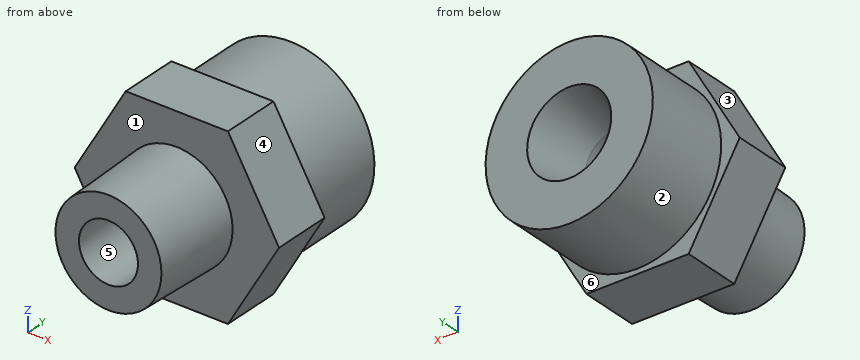
```python
from build123d import *

# Parameters (mm, degrees)
SKETCH1_R           = 9
BOSS_EXTRUDE1_DEPTH = 9.525
SKETCH4_R           = 3.175
CUT_EXTRUDE1_DEPTH  = 3.175
SKETCH5_R           = 3.175
CUT_EXTRUDE2_DEPTH  = 15.224011389
CUT_EXTRUDE2_DRAFT  = 12
BOSS_EXTRUDE3_START = 6.35
SKETCH6_R           = 3.175
BOSS_EXTRUDE3_DEPTH = 6.35
SKETCH7_R           = 6
BOSS_EXTRUDE4_DEPTH = 9.525
BOSS_EXTRUDE4_TAPER = 1.79
SKETCH8_R           = 3.175
CUT_EXTRUDE3_DEPTH  = 30.272053652


with BuildPart() as part:
    # Sketch1 → Boss-Extrude1 (new body)
    with BuildSketch(Plane(origin=(0, 0, 0), x_dir=(1, 0, 0), z_dir=(0, 1, 0))):
        with Locations(Location((0, 0, 0), (0, 0, 90))):
            Circle(SKETCH1_R)
    extrude(amount=BOSS_EXTRUDE1_DEPTH)

    # Sketch4 → Cut-Extrude1 (cut)
    with BuildSketch(Plane.XZ):
        with Locations(Location((0, 0, 0), (0, 0, 270))):
            Circle(SKETCH4_R)
    extrude(amount=-CUT_EXTRUDE1_DEPTH, mode=Mode.SUBTRACT)


with BuildPart() as cut_extrude2_tool:
    # Sketch5 → Cut-Extrude2 (with draft: the straight prism first)
    with BuildSketch(Plane(origin=(0, 3.175, 0), x_dir=(-1, 0, 0), z_dir=(0, -1, 0))):
        with Locations(Location((0, 0, 0), (0, 0, 90))):
            Circle(SKETCH5_R)
    extrude(amount=-CUT_EXTRUDE2_DEPTH)
    # Cut-Extrude2: the draft: its side faces are tilted about the plane it starts from
    cut_extrude2_sides = [cut_extrude2_tool.faces().sort_by_distance(p)[0] for p in [
        (0, 10.787005695, 3.175),
    ]]
    draft(cut_extrude2_sides, Plane(origin=(0, 3.175, 0), x_dir=(-1, 0, 0), z_dir=(0, -1, 0)), CUT_EXTRUDE2_DRAFT)


with BuildPart() as part_1:
    add(part.part)

    # Cut-Extrude2: cut by cut_extrude2_tool
    add(cut_extrude2_tool.part, mode=Mode.SUBTRACT)

    # Sketch6 → Boss-Extrude3 (add)
    with BuildSketch(Plane.XZ.offset(BOSS_EXTRUDE3_START)):
        Polygon((-10.998522628, 0), (-5.499261314, -9.525), (5.499261314, -9.525), (10.998522628, 0), (5.499261314, 9.525), (-5.499261314, 9.525), align=None)
        with Locations(Location((0, 0, 0), (0, 0, 270))):
            Circle(SKETCH6_R, mode=Mode.SUBTRACT)
    extrude(amount=-BOSS_EXTRUDE3_DEPTH)

    # Sketch7 → Boss-Extrude4 (add)
    with BuildSketch(Plane.XZ.offset(6.35)):
        Circle(SKETCH7_R)
    extrude(amount=BOSS_EXTRUDE4_DEPTH, taper=BOSS_EXTRUDE4_TAPER)

    # Sketch8 → Cut-Extrude3 (cut, through all)
    with BuildSketch(Plane.XZ.offset(15.875)):
        with Locations(Location((0, 0, 0), (0, 0, 270))):
            Circle(SKETCH8_R)
    extrude(amount=-CUT_EXTRUDE3_DEPTH, mode=Mode.SUBTRACT)


solid = part_1.part
```
Check sheet for the modelled part. Datum: model origin and axes. Units: mm. Face numbers are marked on the shaded views. A direction names the side the tool comes from. Coordinates: 2 decimals unless noted, no trailing zeros. Loops run counter-clockwise (first coordinate to the right, second up) from the corner with the lowest first, then second, coordinate; pieces in that order, holes last. Notation, with made-up numbers: M 72.25,63.5 L 77.25,63.5 A23 ccw 77.25,97.5 Z; hole C 33,-3.5 d11. An arc over 180 degrees is marked long. Answer as a JSON object with one key per item and string values.
1. Release check for a two-part mould opening along Z. For the marked faces 4, 5 and 6 record: pulls with the +Z half, pulls with the -Z half, needs draft (parallel to the pull), parting line crosses it, or undercut.
Outcome:
{"face 4": "pulls with the +Z half", "face 5": "undercut", "face 6": "needs draft"}
2. Scan lines: L1, parallel to Z at x = 2.75, y = -11.5; L2, parallel to Z at x = -2.5, y = 2.75; L3, parallel to X at y = -7.5, z = 0 (3 decimals). Record each from-to range of solid material in increasing order. Write a range as from..to.
Outcome:
{"L1": "-5.15..-1.59, 1.59..5.15", "L2": "-8.65..-1.96, 1.96..8.65", "L3": "-5.964..-3.175, 3.175..5.964"}
3. Access from +Z, -Z, +X, -X, +Y, -Y to the whole of each face (thin tool, end or side, straight path). Record for the marked faces 1, 2 and 3.
Outcome:
{"face 1": "-Y", "face 2": "+Y", "face 3": "+Z, -X, +Y, -Y"}
4. Sectioned sample at B-B on y = -1.75. Record the cut outline in (x, z) (3 decimals).
Outcome:
{"outline": "M -10.999,0 L -5.499,-9.525 L 5.499,-9.525 L 10.999,0 L 5.499,9.525 L -5.499,9.525 Z; hole C 0,0 d6.35"}
5. Depth check by flat-ended pin: P1, Ø3, axis at x = 5, y = -9.5, coming from the +Z side; P2, Ø4, axis at y = 1, z = -6, coming from the -X side; P3, Ø5, axis at y = 0.5, z = 3, coming from the -X side. Enter the tip coordinate at first touch or a pass-through.
Outcome:
{"P1": "z = 4.75", "P2": "x = -8.53", "P3": "x = -10.68"}
6. Sectioned sample at D-D on x = -8.25. Record the cut outline in (y, z) (3 decimals), and give its area (3 significant figures).
Outcome:
{"outline": "M -6.35,-4.761 L 0,-4.761 L 0,-3.597 L 9.525,-3.597 L 9.525,3.597 L 0,3.597 L 0,4.761 L -6.35,4.761 Z", "area": "129 mm²"}
7. Sectioned sample at C-C on z = -7.75. Record the cut outline in (x, y) (3 decimals), and give its area (3 significant figures).
Outcome:
{"outline": "M -6.524,-6.35 L 6.524,-6.35 L 6.524,0 L 4.576,0 L 4.576,9.525 L -4.576,9.525 L -4.576,0 L -6.524,0 Z", "area": "170 mm²"}
8. Sectioned sample at A-A on x = 0. Record the cut outline in (y, z) (3 decimals), and give its area (3 significant figures).
Outcome:
{"outline": "M -15.875,-5.702 L -6.35,-6 L -6.35,-9.525 L 0,-9.525 L 0,-9 L 9.525,-9 L 9.525,-4.525 L 3.175,-3.175 L -15.875,-3.175 Z; M -15.875,3.175 L 3.175,3.175 L 9.525,4.525 L 9.525,9 L 0,9 L 0,9.525 L -6.35,9.525 L -6.35,6 L -15.875,5.702 Z", "area": "234 mm²"}
